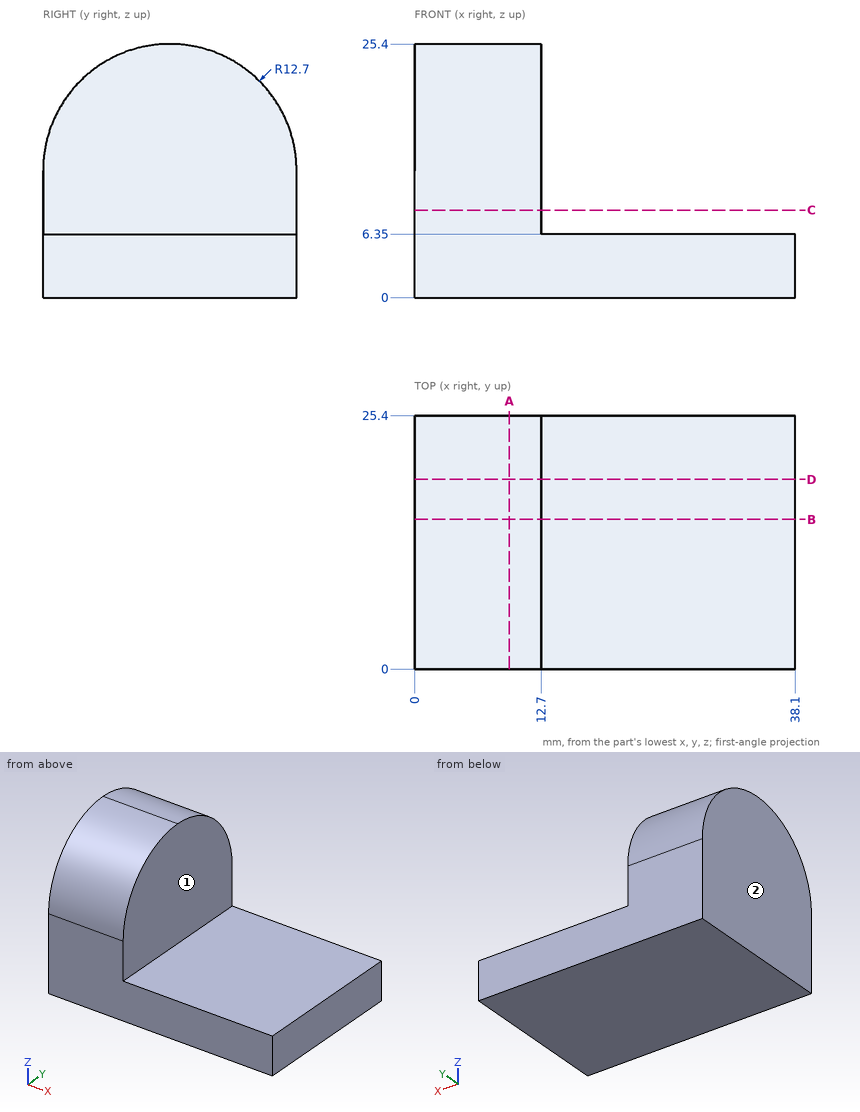
Here's the drawing with two shaded views (mm, measured from the low corner). I have some questions. A direction names the side the tool comes from. Round coordinates to 2 decimals unless told otherwise and drop trailing zeros. Loops run counter-clockwise (first coordinate to the right, second up) from the corner with the lowest first, then second, coordinate; pieces in that order, holes last.
1. Suppose I cut it at D-D, the plane y = 19. Please give me the cut outline in (x, z), and give its area (3 significant figures).
Answers:
outline: (0, 0) - (38.1, 0) - (38.1, 6.35) - (12.7, 6.35) - (12.7, 23.73) - (0, 23.73) - close
area: 463 mm2
2. Suppose I cut it at B-B, the plane y = 15. Please give me the cut outline in (x, z).
Answers:
outline: (0, 0) - (38.1, 0) - (38.1, 6.35) - (12.7, 6.35) - (12.7, 25.19) - (0, 25.19) - close
3. For the marked faces 1 and 2, which set-ups out of +Z, -Z, +X, -X, +Y, -Y let a thin tool reach every point of the face, with its end or its side?
Answers:
face 1: +Z, +X, +Y, -Y
face 2: +Z, -Z, -X, +Y, -Y
4. Will these pins go through, and if not, where does the flat tip stop? pin 1 (2 mm diameter, centred on x = 17.5, y = 6, fed in from +Z); pin 2 (9.5 mm diameter, centred on y = 7, z = 16.5, fed in from +X); pin 3 (5 mm diameter, centred on y = 9, z = 7, fed in from +X).
Answers:
pin 1: stops at z = 6.35
pin 2: stops at x = 12.7
pin 3: stops at x = 38.1
5. Suppose I cut it at A-A, the plane x = 9.5. Please give me the cut outline in (y, z), and give its area (3 significant figures).
Answers:
outline: (0, 0) - (25.4, 0) - (25.4, 12.7) arc R12.7 ccw to (0, 12.7) - close
area: 576 mm2
6. Suppose I cut it at C-C, the plane z = 8.75. Please give me the cut outline in (x, y).
Answers:
outline: (0, 0) - (12.7, 0) - (12.7, 25.4) - (0, 25.4) - close
7. If I drill on probe 1 along Z at (x, y) = (34, 23); probe 2 along X at (y, z) = (21.75, 16.75); probe 3 along Y at (x, z) = (2, 14.75), over which ranges is the centre line in solid material (lowest first)?
Answers:
probe 1: z = 0 to 6.35
probe 2: x = 0 to 12.7
probe 3: y = 0.17 to 25.23
